Here's the drawing with two shaded views (mm, measured from the low corner). I have some questions. Coordinates: 2 decimals unless noted, no trailing zeros. Loops run counter-clockwise (first coordinate to the right, second up) from the corner with the lowest first, then second, coordinate; pieces in that order, holes last. Notation, with made-up numbers: (37, -22) -> (62, -22) arc R14 ccw to (62, -17) -> close; hole circle Ø10 at (-24.5, 81). An arc over 180 degrees is marked (long way). Answer as a JSON object with one key per item and string values. Group by question number.
1) If we mould it in two halves opening along Y, with no side actions, what happens to the marked faces 1, 2 and 3? For each: +Y half, -Y half, draft (parallel to the pull), parting line (faces both ways), or undercut.
2) I want a section at C-C (x = 21.5). Write out the boundary of the cut face in (y, z), then the cut area to 3 significant figures.
3) I'm going to push flat-ended pins straight in: pin 1 (1 mm diameter, centred on y = 25, z = 23.5, fed in from -X); pin 2 (10 mm diameter, centred on x = 18.5, y = 31.5, fed in from +Z). Where does each tip first touch, or does it pass through?
4) I need wall thicknesses on probe 1 along X at (y, z) = (31, 36.5); probe 2 along Y at (x, z) = (7, 39.5) (1 decimal); probe 3 along X at (y, z) = (25, 32). Which ranges of each line are inside material? Lowest first, please. Write a range as [from, to].
5) I want a section at A-A (z = 4). Write out the boundary of the cut face in (x, y), then the cut area to 3 significant figures.
6) I want a section at D-D (y = 23.5). Write out the boundary of the cut face in (x, z).
7) I want a section at B-B (z = 41). Write out the boundary of the cut face in (x, y) (1 decimal).
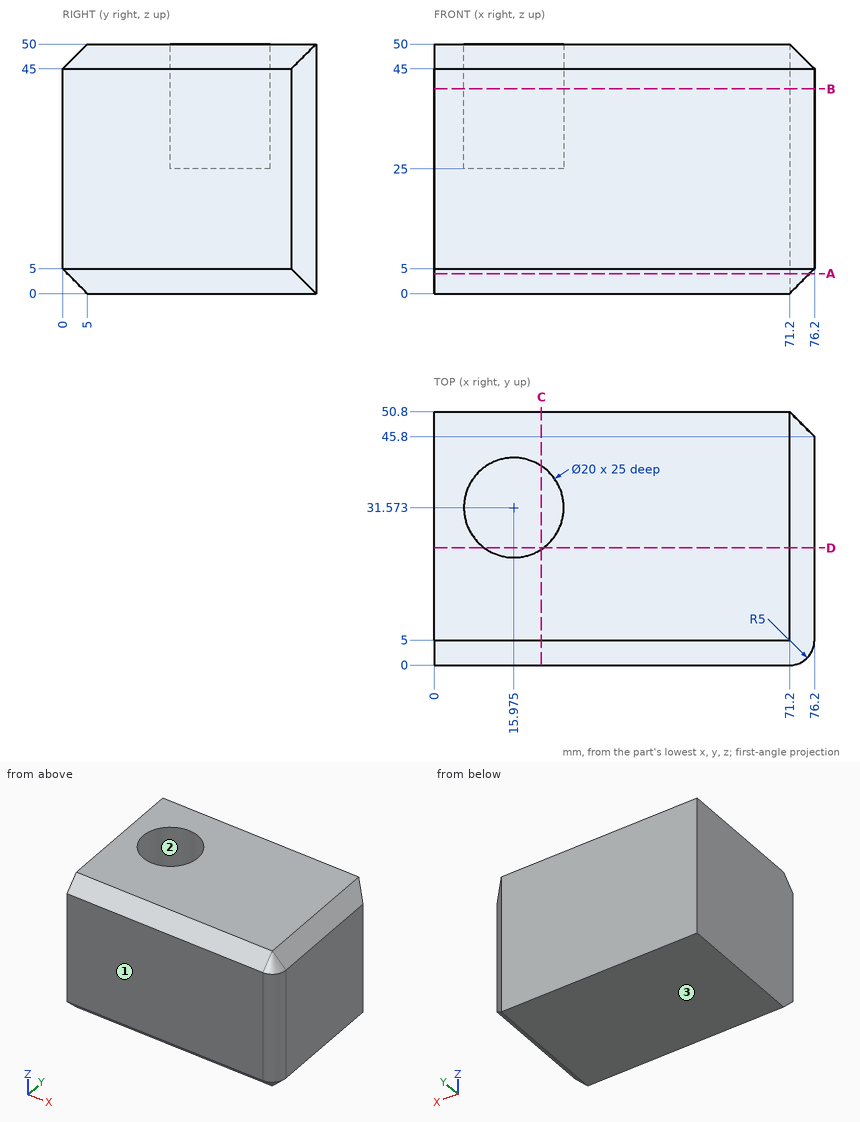
Determined:
{
 "1": {"face 1": "-Y half", "face 2": "undercut", "face 3": "draft"},
 "2": {"outline": "(0, 5) -> (5, 0) -> (50.8, 0) -> (50.8, 50) -> (39.91, 50) -> (39.91, 25) -> (23.24, 25) -> (23.24, 50) -> (5, 50) -> (0, 45) -> close", "area": "2,100 mm^2"},
 "3": {"pin 1": "x = 0", "pin 2": "z = 25"},
 "4": {"probe 1": "[0, 5.99], [25.96, 76.2]", "probe 2": "[0, 27.2], [36, 50.8]", "probe 3": "[0, 8.44], [23.51, 76.2]"},
 "5": {"outline": "(0, 1) -> (71.2, 1) arc R4 ccw to (75.2, 5) -> (75.2, 46.8) -> (71.2, 50.8) -> (0, 50.8) -> close", "area": "3,730 mm^2"},
 "6": {"outline": "(0, 0) -> (71.2, 0) -> (76.2, 5) -> (76.2, 45) -> (71.2, 50) -> (21.88, 50) -> (21.88, 25) -> (10.07, 25) -> (10.07, 50) -> (0, 50) -> close"},
 "7": {"outline": "(0, 0) -> (71.2, 0) arc R5 ccw to (76.2, 5) -> (76.2, 45.8) -> (71.2, 50.8) -> (0, 50.8) -> close; hole circle Ø20 at (16, 31.6)"}
}
